Part print with two shaded views. Sizes in mm from the minimum x, y, z corner. A direction names the side the tool comes from. Round coordinates to 2 decimals unless told otherwise and drop trailing zeros. Loops run counter-clockwise (first coordinate to the right, second up) from the corner with the lowest first, then second, coordinate; pieces in that order, holes last. Notation, with made-up numbers: (88, -5) -> (97, -5) arc R11 ccw to (97, 12) -> close; hole circle Ø9 at (29.25, -13.75). An arc over 180 degrees is marked (long way). Use a Markdown table: item, result. Add a question column.
Item 1: Cut at D-D, the plane y = 7.75. List the corners of the cut face in (x, z).
Item 2: Flat gauge pins, fed straight in: pin 1 (1.8 mm diameter, centred on x = 2.5, y = 21.9, fed in from -Z); pin 2 (8 mm diameter, centred on x = 9.5, z = 12.5, fed in from -Y); pin 3 (8 mm diameter, centred on x = 13, z = 8, fed in from -Y); pin 4 (4 mm diameter, centred on x = 40.5, y = 13, fed in from +Z). Where does each tip first touch, or does it go through?
Item 3: Which spindle directions (+Z, -Z, +X, -X, +Y, -Y) get a long thin tool onto all of the face, cutting with end or side? Do the marked faces 1, 2 and 3. Say none if no direction does.
Item 4: Probe line 1 (Y direction, x = 45.5, z = 1.4); line 2 (Y direction, x = 40.5, z = 0.5); line 3 (Z direction, x = 37.5, y = 7.5). List the from-to ranges inside material, lowest first. Write a range as [from, to].
Item 5: Cut at A-A, the plane x = 45.5. List the corners of the cut face in (y, z), plus the area to 3 significant figures.
Item 6: Cut at C-C, the plane z = 1.25. List the corners of the cut face in (x, y), plus the area to 3 significant figures.
Item 7: Cut at B-B, the plane x = 7.5. List the corners of the cut face in (y, z).
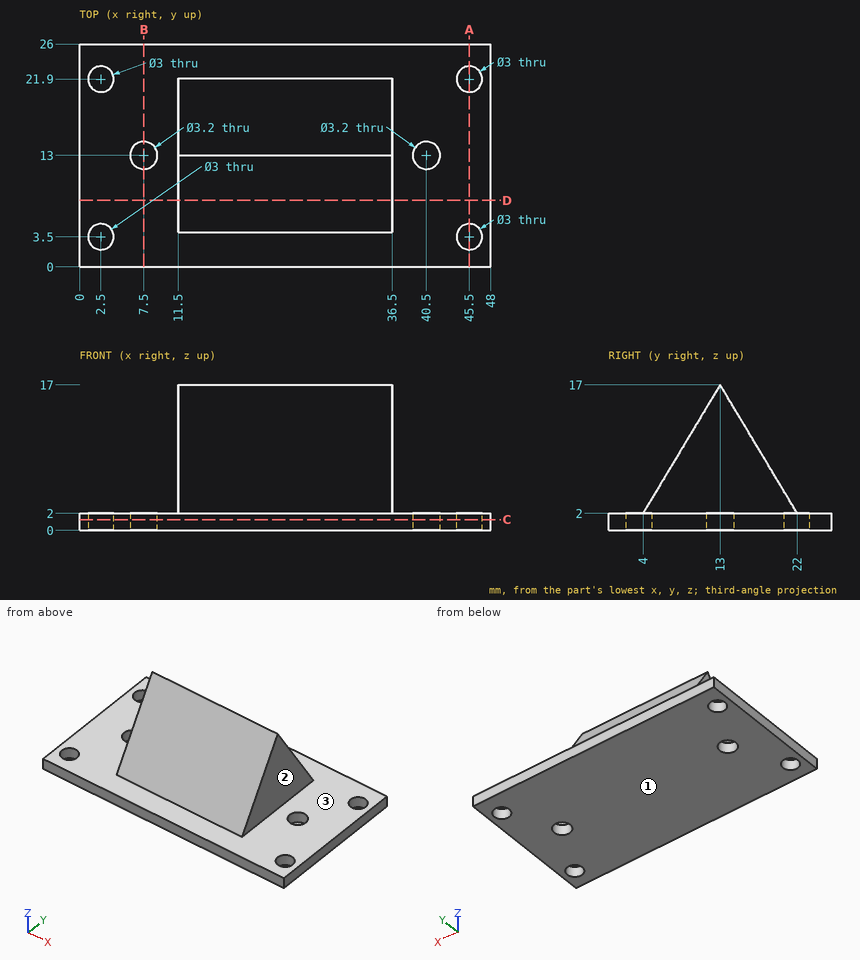
A:
| question | item | result |
|---|---|---|
| 1 | outline | (0, 0) -> (48, 0) -> (48, 2) -> (36.5, 2) -> (36.5, 8.25) -> (11.5, 8.25) -> (11.5, 2) -> (0, 2) -> close |
| 2 | pin 1 | passes through |
| 2 | pin 2 | stops at y = 8.22 |
| 2 | pin 3 | stops at y = 5.2 |
| 2 | pin 4 | stops at z = 2 |
| 3 | face 1 | -Z, +X, -X, +Y, -Y |
| 3 | face 2 | +Z, +X, +Y, -Y |
| 3 | face 3 | +Z |
| 4 | line 1 | y = [0, 2], [5, 20.4], [23.4, 26] |
| 4 | line 2 | y = [0, 11.4], [14.6, 26] |
| 4 | line 3 | z = [0, 2] |
| 5 | outline | (0, 0) -> (2, 0) -> (2, 2) -> (0, 2) -> close; (5, 0) -> (20.4, 0) -> (20.4, 2) -> (5, 2) -> close; (23.4, 0) -> (26, 0) -> (26, 2) -> (23.4, 2) -> close |
| 5 | area | 40.0 mm^2 |
| 6 | outline | (0, 0) -> (48, 0) -> (48, 26) -> (0, 26) -> close; hole circle Ø3 at (2.5, 3.5); hole circle Ø3 at (2.5, 21.9); hole circle Ø3.2 at (7.5, 13); hole circle Ø3.2 at (40.5, 13); hole circle Ø3 at (45.5, 3.5); hole circle Ø3 at (45.5, 21.9) |
| 6 | area | 1,200 mm^2 |
| 7 | outline | (0, 0) -> (11.4, 0) -> (11.4, 2) -> (0, 2) -> close; (14.6, 0) -> (26, 0) -> (26, 2) -> (14.6, 2) -> close |
